from build123d import *

# Parameters (mm, degrees)
SKETCH_1_R          = 1
SKETCH_1_W          = 23
SKETCH_1_H          = 13
EXTRUDE_1_DEPTH     = 1.5
CUT_EXTRUDE_1_DEPTH = 3
FILLET_1_R          = 0.5


with BuildPart() as part:
    # 草图1 → 凸台-拉伸1 (new body, symmetric)
    with BuildSketch(Plane.XY):
        with BuildLine():
            Line((-75, 12.6), (75, 12.6))
            ThreePointArc((75, 12.6), (87.6, 0), (75, -12.6))
            Line((75, -12.6), (-75, -12.6))
            ThreePointArc((-75, -12.6), (-87.6, 0), (-75, 12.6))
        make_face()
        with Locations((-43.55, 0)):
            Circle(SKETCH_1_R, mode=Mode.SUBTRACT)
        with Locations((-70.95, 0)):
            Circle(SKETCH_1_R, mode=Mode.SUBTRACT)
        with Locations((70.95, 0)):
            Circle(SKETCH_1_R, mode=Mode.SUBTRACT)
        with Locations((43.55, 0)):
            Circle(SKETCH_1_R, mode=Mode.SUBTRACT)
        with Locations((-57.25, 0)):
            Rectangle(SKETCH_1_W, SKETCH_1_H, mode=Mode.SUBTRACT)
        with Locations((57.25, 0)):
            Rectangle(SKETCH_1_W, SKETCH_1_H, mode=Mode.SUBTRACT)
    extrude(amount=EXTRUDE_1_DEPTH, both=True)

    # 草图2 → 切除-拉伸1 (cut)
    with BuildSketch(Plane.XY.offset(1.5)):
        with BuildLine():
            Line((44.95, 6.5), (44.55, 6.5))
            ThreePointArc((44.55, 6.5), (43.984314575, 6.265685425), (43.75, 5.7))
            Line((43.75, 5.7), (43.75, 4.1))
            ThreePointArc((43.75, 4.1), (43.984314575, 3.534314575), (44.55, 3.3))
            Line((44.55, 3.3), (45.75, 3.3))
            Line((45.75, 3.3), (45.75, 6.5))
            Line((45.75, 6.5), (68.75, 6.5))
            Line((68.75, 6.5), (68.75, 3.3))
            Line((68.75, 3.3), (69.95, 3.3))
            ThreePointArc((69.95, 3.3), (70.515685425, 3.534314575), (70.75, 4.1))
            Line((70.75, 4.1), (70.75, 5.7))
            ThreePointArc((70.75, 5.7), (70.515685425, 6.265685425), (69.95, 6.5))
            Line((69.95, 6.5), (69.55, 6.5))
            ThreePointArc((69.55, 6.5), (68.984314575, 6.734314575), (68.75, 7.3))
            Line((68.75, 7.3), (68.75, 9.6))
            Line((68.75, 9.6), (45.75, 9.6))
            Line((45.75, 9.6), (45.75, 7.3))
            ThreePointArc((45.75, 7.3), (45.515685425, 6.734314575), (44.95, 6.5))
        make_face()
        with BuildLine():
            Line((44.55, -3.3), (45.75, -3.3))
            Line((45.75, -3.3), (45.75, -6.5))
            Line((45.75, -6.5), (68.75, -6.5))
            Line((68.75, -6.5), (68.75, -3.3))
            Line((68.75, -3.3), (69.95, -3.3))
            ThreePointArc((69.95, -3.3), (70.515685425, -3.534314575), (70.75, -4.1))
            Line((70.75, -4.1), (70.75, -5.7))
            ThreePointArc((70.75, -5.7), (70.515685425, -6.265685425), (69.95, -6.5))
            Line((69.95, -6.5), (69.55, -6.5))
            ThreePointArc((69.55, -6.5), (68.984314575, -6.734314575), (68.75, -7.3))
            Line((68.75, -7.3), (68.75, -9.6))
            Line((68.75, -9.6), (45.75, -9.6))
            Line((45.75, -9.6), (45.75, -7.3))
            ThreePointArc((45.75, -7.3), (45.515685425, -6.734314575), (44.95, -6.5))
            Line((44.95, -6.5), (44.55, -6.5))
            ThreePointArc((44.55, -6.5), (43.984314575, -6.265685425), (43.75, -5.7))
            Line((43.75, -5.7), (43.75, -4.1))
            ThreePointArc((43.75, -4.1), (43.984314575, -3.534314575), (44.55, -3.3))
        make_face()
        with BuildLine():
            Line((-45.75, 3.3), (-45.75, 6.5))
            Line((-45.75, 6.5), (-68.75, 6.5))
            Line((-68.75, 6.5), (-68.75, 3.3))
            Line((-68.75, 3.3), (-69.95, 3.3))
            ThreePointArc((-69.95, 3.3), (-70.515685425, 3.534314575), (-70.75, 4.1))
            Line((-70.75, 4.1), (-70.75, 5.7))
            ThreePointArc((-70.75, 5.7), (-70.515685425, 6.265685425), (-69.95, 6.5))
            Line((-69.95, 6.5), (-69.55, 6.5))
            ThreePointArc((-69.55, 6.5), (-68.984314575, 6.734314575), (-68.75, 7.3))
            Line((-68.75, 7.3), (-68.75, 9.6))
            Line((-68.75, 9.6), (-45.75, 9.6))
            Line((-45.75, 9.6), (-45.75, 7.3))
            ThreePointArc((-45.75, 7.3), (-45.515685425, 6.734314575), (-44.95, 6.5))
            Line((-44.95, 6.5), (-44.55, 6.5))
            ThreePointArc((-44.55, 6.5), (-43.984314575, 6.265685425), (-43.75, 5.7))
            Line((-43.75, 5.7), (-43.75, 4.1))
            ThreePointArc((-43.75, 4.1), (-43.984314575, 3.534314575), (-44.55, 3.3))
            Line((-44.55, 3.3), (-45.75, 3.3))
        make_face()
        with BuildLine():
            Line((-45.75, -7.3), (-45.75, -9.6))
            Line((-45.75, -9.6), (-68.75, -9.6))
            Line((-68.75, -9.6), (-68.75, -7.3))
            ThreePointArc((-68.75, -7.3), (-68.984314575, -6.734314575), (-69.55, -6.5))
            Line((-69.55, -6.5), (-69.95, -6.5))
            ThreePointArc((-69.95, -6.5), (-70.515685425, -6.265685425), (-70.75, -5.7))
            Line((-70.75, -5.7), (-70.75, -4.1))
            ThreePointArc((-70.75, -4.1), (-70.515685425, -3.534314575), (-69.95, -3.3))
            Line((-69.95, -3.3), (-68.75, -3.3))
            Line((-68.75, -3.3), (-68.75, -6.5))
            Line((-68.75, -6.5), (-45.75, -6.5))
            Line((-45.75, -6.5), (-45.75, -3.3))
            Line((-45.75, -3.3), (-44.55, -3.3))
            ThreePointArc((-44.55, -3.3), (-43.984314575, -3.534314575), (-43.75, -4.1))
            Line((-43.75, -4.1), (-43.75, -5.7))
            ThreePointArc((-43.75, -5.7), (-43.984314575, -6.265685425), (-44.55, -6.5))
            Line((-44.55, -6.5), (-44.95, -6.5))
            ThreePointArc((-44.95, -6.5), (-45.515685425, -6.734314575), (-45.75, -7.3))
        make_face()
    extrude(amount=-CUT_EXTRUDE_1_DEPTH, mode=Mode.SUBTRACT)

    # 圆角1
    fillet_1_edges = [part.edges().sort_by_distance(p)[0] for p in [
        (45.75, -3.3, 0),
        (68.75, -3.3, 0),
        (-45.75, 3.3, 0),
        (-68.75, 3.3, 0),
        (-68.75, -3.3, 0),
        (-45.75, -3.3, 0),
        (45.75, 3.3, 0),
        (68.75, 3.3, 0),
    ]]
    fillet(fillet_1_edges, radius=FILLET_1_R)


solid = part.part
Check sheet for the modelled part. Datum: model origin and axes. Units: mm. A direction names the side the tool comes from. Coordinates: 2 decimals unless noted, no trailing zeros. Loops run counter-clockwise (first coordinate to the right, second up) from the corner with the lowest first, then second, coordinate; pieces in that order, holes last. Notation, with made-up numbers: (-11, 57) -> (2, 57) arc R7 ccw to (2, 62) -> close; hole circle Ø1 at (11, -32.75). An arc over 180 degrees is marked (long way). Write item = value, one per line. Start each with the question number.
1. Depth check by flat-ended pin: P1, Ø0.7, axis at y = 8.5, z = 0.5, coming from the -X side; P2, Ø0.8, axis at y = 5, z = -0.5, coming from the -X side; P3, Ø0.8, axis at y = -5.5, z = 0.5, coming from the -X side. Enter the tip coordinate at first touch or a pass-through.
2. Section check B-B on z = 0.3. Give the number of separate pieces and of enclosed holes in the cut face, then the cut area to 3 significant figures.
3. Section check A-A on x = -57.5. Record the cut outline in (y, z).
4. Draft check along X on faces 3 (the flat face through (68.75, 0, 0)), 4 (the cylindrical face through (-87.597, -0.277, 0.021)), 5 (the cylindrical face through (87.597, 0.277, 0.021)). Enter one of: released by +X, released by -X, zero draft, split by the parting line, or undercut.
5. Material ranges on line 1 (Y direction, x = 70.95, z = -0.75); line 2 (X direction, y = 5, z = -0.9); line 3 (X direction, y = 6, z = -1), recorded low to high.
6. Tool access check on faces 1 (the flat face through (-45.75, 0, 0)), 2 (the flat face through (1, 0, -1.5)). Record the directions out of +Z, -Z, +X, -X, +Y, -Y that give a thin tool (end or side, any length) a straight path to the whole face; none if there is none.
Responses:
q1.P1 = -84.61
q1.P2 = -86.73
q1.P3 = -86.52
q2.separate_pieces = 1
q2.enclosed_holes = 6
q2.area = 3,330 mm2
q3.outline = (-12.6, -1.5) -> (-9.6, -1.5) -> (-9.6, 1.5) -> (-12.6, 1.5) -> close; (9.6, -1.5) -> (12.6, -1.5) -> (12.6, 1.5) -> (9.6, 1.5) -> close
q4.face_3 = undercut
q4.face_4 = released by -X
q4.face_5 = released by +X
q5.line_1 = -12.6 to -1, 1 to 12.6
q5.line_2 = -86.57 to -70.75, -43.75 to 43.75, 70.75 to 86.57
q5.line_3 = -86.08 to -70.69, -43.81 to 43.81, 70.69 to 86.08
q6.face_1 = +Z, -Z
q6.face_2 = -Z, +X, -X, +Y, -Y
